Verification items for this drawing (mm, ordinates from the low corner). A direction names the side the tool comes from. Round coordinates to 2 decimals unless told otherwise and drop trailing zeros. Loops run counter-clockwise (first coordinate to the right, second up) from the corner with the lowest first, then second, coordinate; pieces in that order, holes last. Notation, with made-up numbers: (-19.5, 63.25) - (4.5, 63.25) arc R8 cw to (4.5, 74.25) - close; hole circle Ø7 at (-37, 45.5). An arc over 180 degrees is marked (long way). Use a Markdown table: item, result. Add a question column.
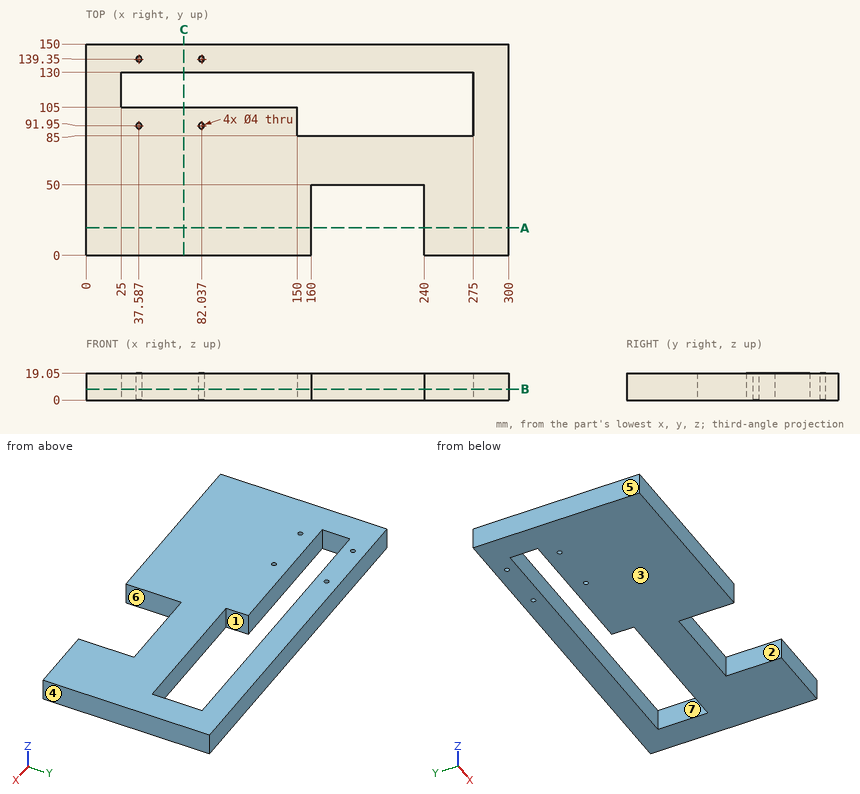
Q1. Thickness scan on line 1 along X through (y, z) = (139.35, 4); line 2 along X through (y, z) = (110, 17); line 3 along Y through (x, z) = (113, 1). Record the ranges inside material, lowest first.
Q2. Set-up check for the marked faces 1, 2 and 3: record each of +Z, -Z, +X, -X, +Y, -Y from which the full face is reachable in a straight line by a thin tool's end or side.
Q3. Go/stop test with flat-tipped pins: pin 1 Ø10 at (x, z) = (225, 5) entering from -Y; pin 2 Ø3.5 at (x, y) = (37.59, 139.35) entering from +Z. Record where each tip stops, or that it passes through.
Q4. Section check B-B on z = 7.75. Record the cut outline in (x, y).
Q5. Release check for a two-part mould opening along X. For the marked faces 4, 5, 6 and 7 record: +X half, -X half, draft (parallel to the pull), parting line (faces both ways), or undercut.
Q6. Section check A-A on y = 19.5. Record the cut outline in (x, z), plus the area to 3 significant figures.
Q7. Section check C-C on x = 69.5. Record the cut outline in (y, z).
Determined:
| question | item | result |
|---|---|---|
| 1 | line 1 | x = 0 to 35.59, 39.59 to 80.04, 84.04 to 300 |
| 1 | line 2 | x = 0 to 25, 275 to 300 |
| 1 | line 3 | y = 0 to 105, 130 to 150 |
| 2 | face 1 | +Z, -Z |
| 2 | face 2 | +Z, -Z, -Y |
| 2 | face 3 | -Z, +X, -X, +Y, -Y |
| 3 | pin 1 | stops at y = 50 |
| 3 | pin 2 | passes through |
| 4 | outline | (0, 0) - (160, 0) - (160, 50) - (240, 50) - (240, 0) - (300, 0) - (300, 150) - (0, 150) - close; hole (25, 105) - (150, 105) - (150, 85) - (275, 85) - (275, 130) - (25, 130) - close; hole circle Ø4 at (37.59, 91.95); hole circle Ø4 at (37.59, 139.35); hole circle Ø4 at (82.04, 91.95); hole circle Ø4 at (82.04, 139.35) |
| 5 | face 4 | +X half |
| 5 | face 5 | -X half |
| 5 | face 6 | undercut |
| 5 | face 7 | undercut |
| 6 | outline | (0, 0) - (160, 0) - (160, 19.05) - (0, 19.05) - close; (240, 0) - (300, 0) - (300, 19.05) - (240, 19.05) - close |
| 6 | area | 4,190 mm² |
| 7 | outline | (0, 0) - (105, 0) - (105, 19.05) - (0, 19.05) - close; (130, 0) - (150, 0) - (150, 19.05) - (130, 19.05) - close |
